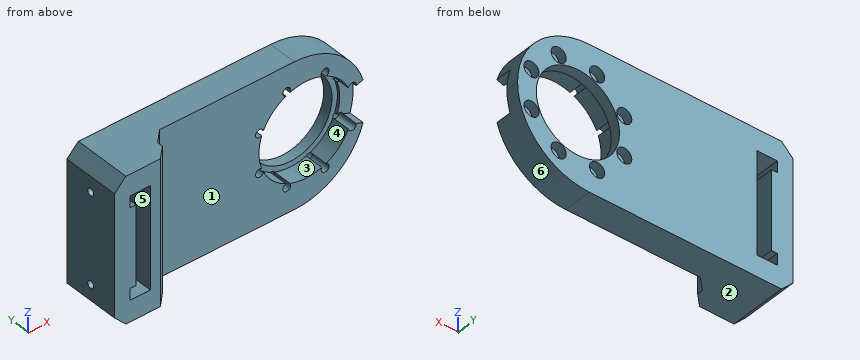
from build123d import *

# Parameters (mm, degrees)
SKETCH1_W                               = 152
SKETCH1_H                               = 100
BOSS_EXTRUDE1_DEPTH                     = 20
BOSS_EXTRUDE2_DEPTH                     = 20
BOSS_EXTRUDE2_DEPTH_BACK                = 20
SKETCH18_W                              = 40
SKETCH18_H                              = 100
SKETCH18_W_2                            = 10
SKETCH18_H_2                            = 70.6
CUT_EXTRUDE3_DEPTH                      = 160.373774505
CUT_EXTRUDE3_DEPTH_BACK                 = 160.373774505
SKETCH19_W                              = 4
SKETCH19_H                              = 8
SKETCH20_R                              = 2.5
CUT_EXTRUDE4_DEPTH                      = 15
CHAMFER1_SIZE                           = 8
CUT_EXTRUDE1_DEPTH                      = 164.095064303
CUT_EXTRUDE1_DEPTH_BACK                 = 164.095064303
SKETCH11_R                              = 29
CUT_EXTRUDE5_DEPTH                      = 11
SKETCH15_R                              = 32.75
CUT_EXTRUDE2_DEPTH                      = 13
CBORE_FOR_M5_HEX_HEAD_BOLT2_D           = 5.5
CBORE_FOR_M5_HEX_HEAD_BOLT2_CBORE_D     = 10.5
CBORE_FOR_M5_HEX_HEAD_BOLT2_CBORE_DEPTH = 6
FILLET1_R                               = 50


with BuildPart() as part:
    # Sketch1 → Boss-Extrude1 (new body)
    with BuildSketch(Plane(origin=(0, 0, 0), x_dir=(1, 0, 0), z_dir=(0, 1, 0))):
        with Locations((-34, 0)):
            Rectangle(SKETCH1_W, SKETCH1_H)
    extrude(amount=BOSS_EXTRUDE1_DEPTH)

    # Sketch18 → Boss-Extrude2 (add, two sides: drawn at the far end of the back side and taken through both)
    with BuildSketch(Plane(origin=(0, 0, 0), x_dir=(1, 0, 0), z_dir=(0, 1, 0)).offset(-BOSS_EXTRUDE2_DEPTH_BACK)):
        with Locations((-130, 0)):
            Rectangle(SKETCH18_W, SKETCH18_H)
        with Locations((-130, 0)):
            Rectangle(SKETCH18_W_2, SKETCH18_H_2, mode=Mode.SUBTRACT)
    extrude(amount=BOSS_EXTRUDE2_DEPTH + BOSS_EXTRUDE2_DEPTH_BACK)

    # Sketch19 → Cut-Extrude3 (cut, two sides: drawn at the far end of the back side and taken through both)
    with BuildSketch(Plane(origin=(0, 0, 0), x_dir=(1, 0, 0), z_dir=(0, 1, 0)).offset(-CUT_EXTRUDE3_DEPTH_BACK)):
        with Locations((-137, -31.3)):
            Rectangle(SKETCH19_W, SKETCH19_H)
        with Locations((-137, 31.3)):
            Rectangle(SKETCH19_W, SKETCH19_H)
    extrude(amount=CUT_EXTRUDE3_DEPTH + CUT_EXTRUDE3_DEPTH_BACK, mode=Mode.SUBTRACT)

    # Sketch20 → Cut-Extrude4 (cut)
    with BuildSketch(Plane.ZY.offset(150)):
        with Locations((-31.3, 0)):
            Circle(SKETCH20_R)
        with Locations((31.3, 0)):
            Circle(SKETCH20_R)
    extrude(amount=-CUT_EXTRUDE4_DEPTH, mode=Mode.SUBTRACT)

    # Chamfer1
    chamfer1_edges = [part.edges().sort_by_distance(p)[0] for p in [
        (-110, -20, 0),
        (-150, 0, 50),
        (-150, 0, -50),
        (-110, 0, 0),
    ]]
    chamfer(chamfer1_edges, length=CHAMFER1_SIZE)

    # Sketch11 → Cut-Extrude1 (cut, two sides: drawn at the far end of the back side and taken through both)
    with BuildSketch(Plane(origin=(0, 20, 0), x_dir=(1, 0, 0), z_dir=(0, 1, 0)).offset(-CUT_EXTRUDE1_DEPTH_BACK)):
        with Locations(Location((0, 0, 0), (0, 0, 90))):
            Circle(SKETCH11_R)
    extrude(amount=CUT_EXTRUDE1_DEPTH + CUT_EXTRUDE1_DEPTH_BACK, mode=Mode.SUBTRACT)

    # Sketch21 → Cut-Extrude5 (cut)
    with BuildSketch(Plane(origin=(0, 0, 0), x_dir=(1, 0, 0), z_dir=(0, 1, 0))):
        Polygon((0, 0), (52.866493453, -19.241830007), (52.866493453, 19.241830007), align=None)
    extrude(amount=CUT_EXTRUDE5_DEPTH, mode=Mode.SUBTRACT)

    # Sketch15 → Cut-Extrude2 (cut)
    with BuildSketch(Plane(origin=(0, 0, 0), x_dir=(1, 0, 0), z_dir=(0, 1, 0))):
        with Locations(Location((0, 0, 0), (0, 0, 20))):
            Circle(SKETCH15_R)
    extrude(amount=CUT_EXTRUDE2_DEPTH, mode=Mode.SUBTRACT)

    # CBORE for M5 Hex Head Bolt2 (through all)
    with Locations(Plane(origin=(-32.335783638, 20, -13.393920133), x_dir=(0, 0, 1), z_dir=(0, 1, 0))):
        with Locations((0, 0), (-18.941863505, 18.941863505), (-18.941863505, 45.729703771), (0, 64.671567276), (26.787840266, 64.671567276), (45.729703771, 45.729703771), (45.729703771, 18.941863505), (26.787840266, 0)):
            CounterBoreHole(CBORE_FOR_M5_HEX_HEAD_BOLT2_D / 2, CBORE_FOR_M5_HEX_HEAD_BOLT2_CBORE_D / 2, CBORE_FOR_M5_HEX_HEAD_BOLT2_CBORE_DEPTH)

    # Fillet1
    fillet1_edges = [part.edges().sort_by_distance(p)[0] for p in [
        (42, 10, -50),
        (42, 10, 50),
    ]]
    fillet(fillet1_edges, radius=FILLET1_R - 0.0001)  # a hair under: the kernel refuses the full size


solid = part.part
Design review of the part built by this model. Coordinates are the model's own, in mm. Face numbers are marked on the shaded views. A direction names the side the tool comes from. Give positions to 0.01 mm unless a question says otherwise; leave off trailing zeros. Loops run counter-clockwise (first coordinate to the right, second up) from the corner with the lowest first, then second, coordinate; pieces in that order, holes last. Notation, with made-up numbers: M -30.5,6.5 L -4.5,6.5 A21 ccw -4.5,39.5 Z; hole C 0.25,46 d6. An arc over 180 degrees is marked long. Write item = value, one per line.
Q1. We need section C-C (z = 40). Give the boundary of the cut face in (x, y), plus the area to 3 significant figures.
Output values:
outline = M -150,-20 L -118,-20 L -110,-12 L -110,-8 L -102,0 L 22,0 L 22,20 L -150,20 Z
area = 4,240 mm^2
Q2. For the marked faces 4, 5 and 6, list the 3-axis set-ups (+Z, -Z, +X, -X, +Y, -Y) from which the entire face can be reached by the end or side of a thin tool; tool diameter is ignored.
Output values:
face_4 = -Y
face_5 = +Y, -Y
face_6 = -Z, +X, +Y, -Y
Q3. To check wall thickness, follow line 1 (X direction, y = 15.5, z = -24.5); line 2 (Z direction, x = -131, y = -15.5); line 3 (Z direction, x = 29.5, y = 16.5). State the ranges of each line that lie inside material, in increasing order. Write a range as [from, to].
Output values:
line_1 = [-150, -135], [-125, -15.52], [15.52, 35.59]
line_2 = [-50, -35.3], [35.3, 50]
line_3 = [-33.07, -17.81], [-8.98, 8.98], [17.81, 33.07]
Q4. We need section B-B (x = 0). Give the boundary of the cut face in (y, z), plus the area to 3 significant figures.
Output values:
outline = M 0,-49.36 L 20,-49.36 L 20,-29 L 13,-29 L 13,-32.75 L 0,-32.75 Z; M 0,32.75 L 13,32.75 L 13,29 L 20,29 L 20,49.36 L 0,49.36 Z
area = 717 mm^2
Q5. Insertion check: pin 1 (4 mm diameter, centred on y = 13.5, z = 23, fed in from +X); pin 2 (5 mm diameter, centred on x = -34, z = 15.5, fed in from +Y); pin 3 (12 mm diameter, centred on x = -13.39, z = 32.34, fed in from -Y); pin 4 (8.5 mm diameter, centred on x = 29.5, z = -15, fed in from +Y). Each pin has a flat end and moves straight along its axis. Give the tip position at first contact, or say it passes through.
Output values:
pin_1 = 37.38
pin_2 = 14
pin_3 = 0
pin_4 = 20
Q6. Draft analysis for pull direction Z (two halves, no side actions). For the marked faces 1, 2 and 3, state which applies: +Z half, -Z half, draft (parallel to the pull), parting line (faces both ways), or undercut.
Output values:
face_1 = draft
face_2 = -Z half
face_3 = undercut
